from build123d import *

# Parameters (mm, degrees)
COLUMN_CIRCULAR_PATTERN_CUT_COUNT = 9


with BuildPart() as part:
    # Sketch1 → Main Support Pole (revolve)
    with BuildSketch(Plane.XY, mode=Mode.PRIVATE) as main_support_pole_sk:
        Polygon((0, 0), (0, 26.2), (3.5, 26.2), (3.5, 23.35), (3.5, 21.35), (3, 20.85), (3, 5.35), (3.5, 4.85), (3.5, 2.85), (3.5, 0), align=None)
    revolve(main_support_pole_sk.sketch.rotate(Axis((0, 26.2, 0), (0, 1, 0)), 90), axis=Axis((0, 26.2, 0), (0, 1, 0)))

    # Sketch2 → Column Cut (revolve, cut)
    with BuildSketch(Plane(origin=(0, 0, 0), x_dir=(0, 0, -1), z_dir=(1, 0, 0))):
        with BuildLine():
            Line((3, 19.85), (3, 6.35))
            ThreePointArc((3, 6.35), (2.752512627, 6.452512627), (2.65, 6.7))
            Line((2.65, 6.7), (2.65, 19.5))
            ThreePointArc((2.65, 19.5), (2.752512627, 19.747487373), (3, 19.85))
        make_face()
    column_cut = revolve(axis=Axis((0, 19.85, -3), (0, 1, 0)), mode=Mode.SUBTRACT)

    # Column Circular Pattern Cut: Column Cut ×9 about axis
    column_circular_pattern_cut_axis = Axis((0, 0, 0), (0, 1, 0))
    for i in range(1, COLUMN_CIRCULAR_PATTERN_CUT_COUNT):
        add(column_cut.rotate(column_circular_pattern_cut_axis, i * 360 / COLUMN_CIRCULAR_PATTERN_CUT_COUNT), mode=Mode.SUBTRACT)


solid = part.part
Check sheet for the modelled part. Datum: model origin and axes. Units: mm. Give positions to 0.01 mm unless a question says otherwise; leave off trailing zeros. Loops run counter-clockwise (first coordinate to the right, second up) from the corner with the lowest first, then second, coordinate; pieces in that order, holes last. Notation, with made-up numbers: M 1,31.5 L 11,31.5 A31 cw 11,62.5 Z; hole C -38.5,65 d8. An arc over 180 degrees is marked long. Answer as a JSON object with one key per item and string values. Group by question number.
Q1. Material ranges on line 1 along Z through (x, y) = (0, 14.75); line 2 along X through (y, z) = (16.5, -2.25); line 3 along Y through (x, z) = (-1, -3), recorded low to high. Write a range as [from, to].
Q2. Cross-section at A-A on x = 0. Record the cut outline in (y, z).
Q3. Release check for a two-part mould opening along Y. For faces 1 (the cylindrical face through (3.105, 2.459, -1.615)), 2 (the flat face through (0, 26.2, 0)), 3 (the cylindrical face through (-0.9, 12.99, -2.86)), 4 (the flat face through (0, 0, 0)) record: released by +Y, released by -Y, zero draft, split by the parting line, or undercut.
Q4. Cross-section at B-B on y = 2.5. Record the cut outline in (x, z), then the cut area to 3 significant figures.
Q5. Go/stop test with a flat-tipped pin: P1, Ø3, axis at y = 10.5, z = -1, coming from the +X side. Record where the tip stops, or that it passes through.
Evaluation:
{
 "1": {"line 1": "z = [-2.65, 3]", "line 2": "x = [-1.58, 1.58]", "line 3": "y = [0, 5.19], [21.01, 26.2]"},
 "2": {"outline": "M 0,-3.5 L 4.85,-3.5 L 5.35,-3 L 6.35,-3 A0.35 cw 6.7,-2.65 L 19.5,-2.65 A0.35 cw 19.85,-3 L 20.85,-3 L 21.35,-3.5 L 26.2,-3.5 L 26.2,3.5 L 21.35,3.5 L 20.85,3 L 5.35,3 L 4.85,3.5 L 0,3.5 Z"},
 "3": {"face 1": "zero draft", "face 2": "released by +Y", "face 3": "undercut", "face 4": "released by -Y"},
 "4": {"outline": "C 0,0 d7", "area": "38.5 mm2"},
 "5": {"P1": "stops at x = 3"}
}
